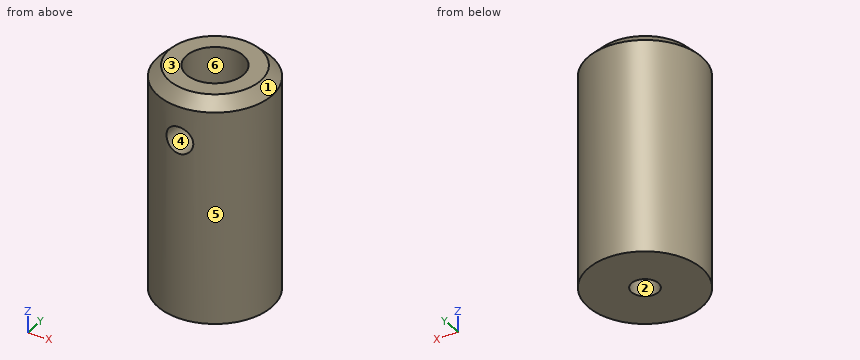
```python
from build123d import *

# Parameters (mm, degrees)
F0_R     = 12.7
F0_R_2   = 6.35
F1_DEPTH = 50
F0_R_3   = 3
F2_DEPTH = 10.8
F3_SIZE  = 2.5
F4_R     = 3
F5_DEPTH = 25


with BuildPart() as f1:
    # F0 (on Top) → F1 (new body)
    with BuildSketch(Plane.XY):
        Circle(F0_R)
        Circle(F0_R_2, mode=Mode.SUBTRACT)
    extrude(amount=F1_DEPTH)

    # F0 (on Top) → F2 (join)
    with BuildSketch(Plane.XY):
        Circle(F0_R_2)
        Circle(F0_R_3, mode=Mode.SUBTRACT)
    extrude(amount=F2_DEPTH)

    # F3
    f3_edges = [f1.edges().sort_by_distance(p)[0] for p in [
        (-12.7, 0, 50),
    ]]
    chamfer(f3_edges, length=F3_SIZE)

    # F4 (on Front) → F5 (cut)
    with BuildSketch(Plane.XZ):
        with Locations((0, 40)):
            Circle(F4_R)
    extrude(amount=F5_DEPTH, mode=Mode.SUBTRACT)


solid = f1.part
```
Verification items for the finished model (mm, model axes). Face numbers are marked on the shaded views. A direction names the side the tool comes from. Coordinates: 2 decimals unless noted, no trailing zeros. Loops run counter-clockwise (first coordinate to the right, second up) from the corner with the lowest first, then second, coordinate; pieces in that order, holes last. Notation, with made-up numbers: (-30, 67) -> (24, 67) arc R16 cw to (24, 76) -> close; hole circle Ø5 at (51, 20.5). An arc over 180 degrees is marked (long way). Answer in a Markdown table with one row per item.
1) Section check D-D (z = 29). Record the cut outline in (x, y), and give its area (3 significant figures).
The answers:
| item | result |
|---|---|
| outline | circle Ø25.4 at (0, 0); hole circle Ø12.7 at (0, 0) |
| area | 380 mm2 |
2) Section check C-C (z = 3). Record the cut outline in (x, y).
The answers:
| item | result |
|---|---|
| outline | circle Ø25.4 at (0, 0); hole circle Ø6 at (0, 0) |
3) Draft check along X on the marked faces 1, 2 and 3. Enter one of: released by +X, released by -X, zero draft, split by the parting line, or undercut.
The answers:
| item | result |
|---|---|
| face 1 | split by the parting line |
| face 2 | undercut |
| face 3 | zero draft |
4) Depth check by flat-ended pin: P1, Ø4, axis at x = -3, y = 2, coming from the +Z side; P2, Ø4, axis at x = -2.5, z = 14, coming from the -Y side; P3, Ø1, axis at x = -5, z = 11, coming from the -Y side. Enter the tip coordinate at first touch or a pass-through.
The answers:
| item | result |
|---|---|
| P1 | stops at z = 10.8 |
| P2 | stops at y = -12.69 |
| P3 | stops at y = -11.88 |
5) Section check A-A (x = 0). Record the cut outline in (y, z).
The answers:
| item | result |
|---|---|
| outline | (-12.7, 0) -> (-3, 0) -> (-3, 10.8) -> (-6.35, 10.8) -> (-6.35, 37) -> (-12.7, 37) -> close; (-12.7, 43) -> (-6.35, 43) -> (-6.35, 50) -> (-10.2, 50) -> (-12.7, 47.5) -> close; (3, 0) -> (12.7, 0) -> (12.7, 47.5) -> (10.2, 50) -> (6.35, 50) -> (6.35, 10.8) -> (3, 10.8) -> close |
6) Scan lines: line 1 along Z through (x, y) = (-0.25, -6.5); line 2 along Y through (x, z) = (0, 8.75); line 3 along X through (y, z) = (0.25, 19). Record each from-to range of solid material in increasing order. Write a range as from..to.
The answers:
| item | result |
|---|---|
| line 1 | z = 0..37.01, 42.99..50 |
| line 2 | y = -12.7..-3, 3..12.7 |
| line 3 | x = -12.7..-6.35, 6.35..12.7 |
7) Section check B-B (y = 0). Record the cut outline in (x, z), and give its area (3 significant figures).
The answers:
| item | result |
|---|---|
| outline | (-12.7, 0) -> (-3, 0) -> (-3, 10.8) -> (-6.35, 10.8) -> (-6.35, 50) -> (-10.2, 50) -> (-12.7, 47.5) -> close; (3, 0) -> (12.7, 0) -> (12.7, 47.5) -> (10.2, 50) -> (6.35, 50) -> (6.35, 10.8) -> (3, 10.8) -> close |
| area | 701 mm2 |
8) Access from +Z, -Z, +X, -X, +Y, -Y to the whole of each face (thin tool, end or side, straight path). Record for the marked faces 4, 5 and 6.
The answers:
| item | result |
|---|---|
| face 4 | -Y |
| face 5 | +Z, -Z |
| face 6 | +Z |
